CAD build for the part. Positions are in the model's coordinates, mm. A direction names the side the tool comes from. Give positions to 0.01 mm unless a question says otherwise; leave off trailing zeros. Loops run counter-clockwise (first coordinate to the right, second up) from the corner with the lowest first, then second, coordinate; pieces in that order, holes last. Notation, with made-up numbers: (48.25, 23) -> (53.25, 23) arc R15 cw to (53.25, 35) -> close; hole circle Ø8 at (56, 56.5). An arc over 180 degrees is marked (long way). Use one line per item in the form item = value.
```python
from build123d import *

# Parameters (mm, degrees)
BOSS_EXTRU_1_DEPTH                                = 20
CHAMBRAGE_POUR_VIS_SIX_PANS_CREUX_M41_D           = 4.5
CHAMBRAGE_POUR_VIS_SIX_PANS_CREUX_M41_DEPTH       = 11.55
CHAMBRAGE_POUR_VIS_SIX_PANS_CREUX_M41_CBORE_D     = 8
CHAMBRAGE_POUR_VIS_SIX_PANS_CREUX_M41_CBORE_DEPTH = 1
ESQUISSE6_W                                       = 20.2
ESQUISSE6_H                                       = 20
ENL_V_MAT_EXTRU_1_DEPTH                           = 3
ESQUISSE14_W                                      = 30.8
ESQUISSE14_H                                      = 2.5
BOSS_EXTRU_3_DEPTH                                = 40
CHAMBRAGE_POUR_VIS_SIX_PANS_CREUX_M31_D           = 3.4
CHAMBRAGE_POUR_VIS_SIX_PANS_CREUX_M31_CBORE_D     = 6.5
CHAMBRAGE_POUR_VIS_SIX_PANS_CREUX_M31_CBORE_DEPTH = 3.4
CHANFREIN1_SIZE                                   = 6.25


with BuildPart() as part:
    # Base → Boss.-Extru.1 (new, symmetric)
    with BuildSketch(Plane(origin=(0, 0, 0), x_dir=(1, 0, 0), z_dir=(0, 1, 0))):
        Polygon((-3.85, -2.4), (-3.85, 2.4), (-10.1, 2.4), (-10.1, 10.1), (-2.4, 10.1), (-2.4, 3.85), (2.4, 3.85), (2.4, 10.1), (10.1, 10.1), (10.1, 2.4), (3.85, 2.4), (3.85, -2.4), (10.1, -2.4), (10.1, -6.25), (15.4, -6.25), (15.4, 15.4), (-15.4, 15.4), (-15.4, -6.25), (-10.1, -6.25), (-10.1, -2.4), align=None)
    extrude(amount=BOSS_EXTRU_1_DEPTH, both=True)

    # Chambrage pour vis à six pans creux M41
    with Locations(Plane(origin=(15.4, 0, 0), x_dir=(0, 0, -1), z_dir=(1, 0, 0))):
        with Locations((0, 0)):
            chambrage_pour_vis_six_pans_creux_m41 = CounterBoreHole(CHAMBRAGE_POUR_VIS_SIX_PANS_CREUX_M41_D / 2, CHAMBRAGE_POUR_VIS_SIX_PANS_CREUX_M41_CBORE_D / 2, CHAMBRAGE_POUR_VIS_SIX_PANS_CREUX_M41_CBORE_DEPTH, depth=CHAMBRAGE_POUR_VIS_SIX_PANS_CREUX_M41_DEPTH)

    # Symétrie1: Chambrage pour vis à six pans creux M41 across plane
    add(chambrage_pour_vis_six_pans_creux_m41.mirror(Plane(origin=(0, 0, 0), x_dir=(0, 0, 1), z_dir=(1, 0, 0))), mode=Mode.SUBTRACT)

    # Esquisse6 → Enlèv. mat.-Extru.1 (cut, symmetric)
    with BuildSketch(Plane.XY):
        Rectangle(ESQUISSE6_W, ESQUISSE6_H)
    extrude(amount=ENL_V_MAT_EXTRU_1_DEPTH, both=True, mode=Mode.SUBTRACT)

    # Esquisse14 → Boss.-Extru.3 (add)
    with BuildSketch(Plane.XZ.offset(20)):
        with Locations((0, -16.65)):
            Rectangle(ESQUISSE14_W, ESQUISSE14_H)
    extrude(amount=-BOSS_EXTRU_3_DEPTH)

    # Chambrage pour vis à six pans creux M31 (through all)
    with Locations(Plane.XY.offset(-10.1)):
        with Locations((-6.717514421, 6.717514421), (-6.717514421, -6.717514421), (6.717514421, 6.717514421), (6.717514421, -6.717514421)):
            CounterBoreHole(CHAMBRAGE_POUR_VIS_SIX_PANS_CREUX_M31_D / 2, CHAMBRAGE_POUR_VIS_SIX_PANS_CREUX_M31_CBORE_D / 2, CHAMBRAGE_POUR_VIS_SIX_PANS_CREUX_M31_CBORE_DEPTH)

    # Chanfrein1
    chanfrein1_edges = [part.edges().sort_by_distance(p)[0] for p in [
        (3.85, -10, 0),
        (-3.85, -10, 0),
    ]]
    chamfer(chanfrein1_edges, length=CHANFREIN1_SIZE - 0.0001)  # a hair under: the kernel refuses the full size


solid = part.part
```
1. Cut at A-A, the plane y = 0. Write the cut outline in (x, z), then the cut area to 3 significant figures.
Result sheet:
outline = (-15.4, -17.9) -> (15.4, -17.9) -> (15.4, -4) -> (14.4, -4) -> (14.4, -2.25) -> (10.1, -2.25) -> (10.1, -10.1) -> (2.4, -10.1) -> (2.4, -3.85) -> (-2.4, -3.85) -> (-2.4, -10.1) -> (-10.1, -10.1) -> (-10.1, -2.25) -> (-14.4, -2.25) -> (-14.4, -4) -> (-15.4, -4) -> close; (-15.4, 4) -> (-14.4, 4) -> (-14.4, 2.25) -> (-10.1, 2.25) -> (-10.1, 6.25) -> (-15.4, 6.25) -> close; (10.1, 2.25) -> (14.4, 2.25) -> (14.4, 4) -> (15.4, 4) -> (15.4, 6.25) -> (10.1, 6.25) -> close
area = 389 mm^2
2. Cut at D-D, the plane y = 11. Write the cut outline in (x, z).
Result sheet:
outline = (-15.4, -17.9) -> (15.4, -17.9) -> (15.4, 6.25) -> (10.1, 6.25) -> (10.1, 2.4) -> (3.85, 2.4) -> (3.85, -2.4) -> (10.1, -2.4) -> (10.1, -10.1) -> (2.4, -10.1) -> (2.4, -3.85) -> (-2.4, -3.85) -> (-2.4, -10.1) -> (-10.1, -10.1) -> (-10.1, -2.4) -> (-3.85, -2.4) -> (-3.85, 2.4) -> (-10.1, 2.4) -> (-10.1, 6.25) -> (-15.4, 6.25) -> close
3. Drop flat-ended pins along their axis: P1, Ø3, axis at x = -3.5, y = -11.5, coming from the +Z side; P2, Ø7, axis at x = 6.5, y = -16.5, coming from the +Z side; P3, Ø6, axis at y = 0, z = 0, coming from the +X side. Give the stop position or say it passes through.
Result sheet:
P1 = -3.85
P2 = 2.4
P3 = 14.4
4. Cut at B-B, the plane z = -7. Write the cut outline in (x, y).
Result sheet:
outline = (-15.4, -20) -> (-10.1, -20) -> (-10.1, 20) -> (-15.4, 20) -> close; (-2.4, -20) -> (2.4, -20) -> (2.4, 20) -> (-2.4, 20) -> close; (10.1, -20) -> (15.4, -20) -> (15.4, 20) -> (10.1, 20) -> close
5. Mould opens along X. For faces 4 (the cylindrical face through (12.22, 2.23, -0.29)), 5 (the flat face through (14.4, -2, -2)), 6 (the flat face through (-8, -16, 2.4)) say: pulls with the +X half, pulls with the -X half, needs draft (parallel to the pull), parting line crosses it, or undercut.
Result sheet:
face_4 = needs draft
face_5 = pulls with the +X half
face_6 = undercut
6. Tool access for faces 1 (the flat face through (-3.85, -18, 0)), 2 (the flat face through (-8, -16, -2.4)), 3 (the cylindrical face through (-9.297, -8.695, -11.776)): list every direction of +Z, -Z, +X, -X, +Y, -Y with a clear straight run to the whole face (end or side of a thin tool).
Result sheet:
face_1 = +Z, +Y, -Y
face_2 = +Y, -Y
face_3 = +Z
7. Cut at C-C, the plane z = 0. State how many separate pieces and enclosed holes the cut face has, then the cut area to 3 significant figures.
Result sheet:
separate_pieces = 4
enclosed_holes = 0
area = 580 mm^2
8. Drill centre lines: line 1 (X direction, y = 12, z = -9.75); line 2 (Z direction, x = 9.5, y = -18); line 3 (Y direction, x = 14.8, z = 0). Where is each one in solid material? Low to high.
Result sheet:
line_1 = -15.4 to -10.1, -2.4 to 2.4, 10.1 to 15.4
line_2 = -17.9 to -10.1, -2.4 to 2.4
line_3 = -20 to -4, 4 to 20
